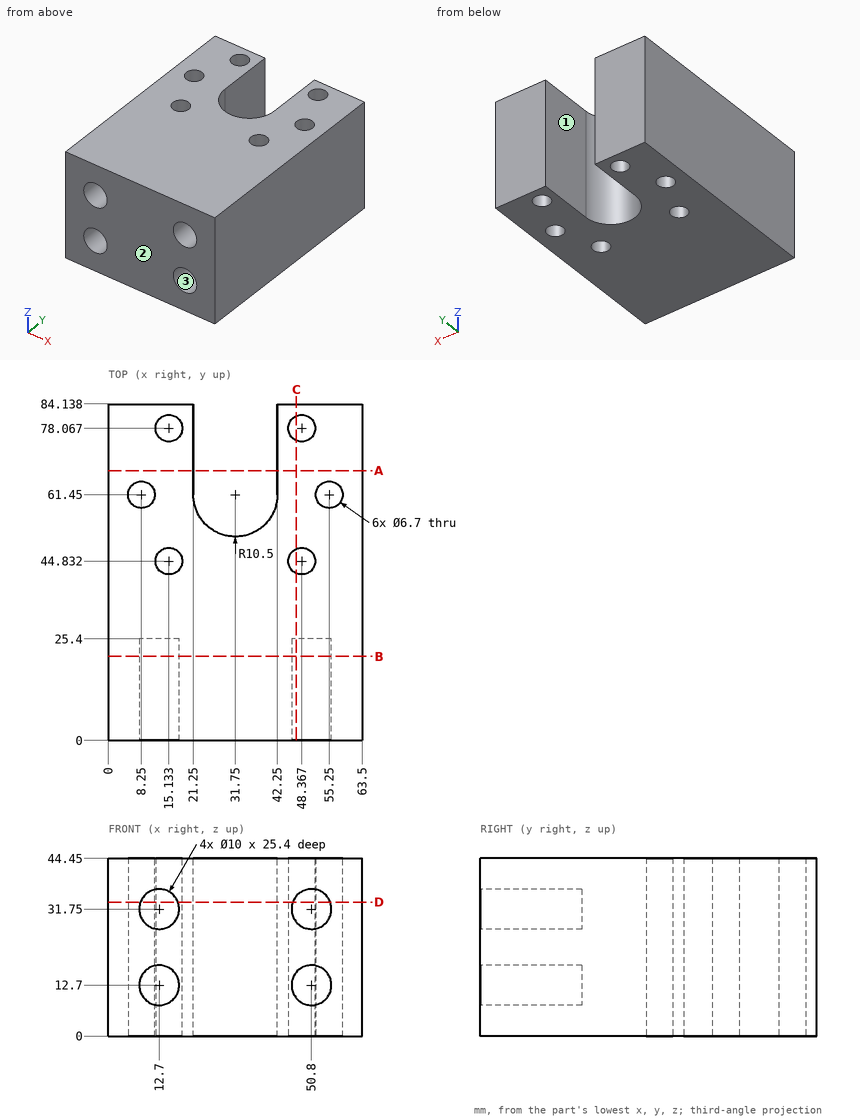
For this review, use the dimensioned drawing (mm, ordinates from the lowest corner) and the shaded views. A direction names the side the tool comes from. Coordinates: 2 decimals unless noted, no trailing zeros. Order: outer loops, then holes, each group sorted by start corner. A loop starts at its lowest first (then second) coordinate and runs counter-clockwise, first axis right, second up. Notation, with made-up numbers: (23, 46.25) - (28, 46.25) arc R14 cw to (28, 52.25) - close; hole circle Ø1 at (44, 7.5). An arc over 180 degrees is marked (long way). Answer as a JSON object with one key per item and string values. Group by question number.
1. Clearance check with flat-ended pins moving along their axes: P1, Ø10.5, axis at x = 48.37, y = 44.83, coming from the -Z side; P2, Ø5, axis at x = 51, z = 30, coming from the -Y side. State where each tip first meets the part, or that it passes through.
2. For probe 1 along Z at (x, y) = (12.7, 8.25); probe 2 along X at (y, z) = (63, 40); probe 3 along Y at (x, z) = (55.5, 3), list the stretches that pass through material, from the lowest coordinate up.
3. We need section B-B on y = 21. State the section outline as (x, z) points, then the cut area to 3 significant figures.
4. We need section C-C on x = 47. Give the number of separate pieces and of enclosed holes in the cut face, then the cut area to 3 significant figures.
5. We need section D-D on z = 33.5. State the section outline as (x, y) points.
6. We need section A-A on y = 67.5. State the section outline as (x, z) points.
7. For the marked faces 1, 2 and 3, list the 3-axis set-ups (+Z, -Z, +X, -X, +Y, -Y) from which the entire face can be reached by the end or side of a thin tool; tool diameter is ignored.
Final values:
{
 "1": {"P1": "z = 0", "P2": "y = 25.4"},
 "2": {"probe 1": "0 to 7.7, 17.7 to 26.75, 36.75 to 44.45", "probe 2": "0 to 5.28, 11.22 to 21.25, 42.25 to 52.28, 58.22 to 63.5", "probe 3": "0 to 58.11, 64.79 to 84.14"},
 "3": {"outline": "(0, 0) - (63.5, 0) - (63.5, 44.45) - (0, 44.45) - close; hole circle Ø10 at (12.7, 12.7); hole circle Ø10 at (12.7, 31.75); hole circle Ø10 at (50.8, 12.7); hole circle Ø10 at (50.8, 31.75)", "area": "2,510 mm²"},
 "4": {"separate pieces": "3", "enclosed holes": "0", "area": "2,870 mm²"},
 "5": {"outline": "(0, 0) - (8.02, 0) - (8.02, 25.4) - (17.38, 25.4) - (17.38, 0) - (46.12, 0) - (46.12, 25.4) - (55.48, 25.4) - (55.48, 0) - (63.5, 0) - (63.5, 84.14) - (42.25, 84.14) - (42.25, 61.45) arc R10.5 cw to (21.25, 61.45) - (21.25, 84.14) - (0, 84.14) - close; hole circle Ø6.7 at (8.25, 61.45); hole circle Ø6.7 at (15.13, 44.83); hole circle Ø6.7 at (15.13, 78.07); hole circle Ø6.7 at (48.37, 44.83); hole circle Ø6.7 at (48.37, 78.07); hole circle Ø6.7 at (55.25, 61.45)"},
 "6": {"outline": "(0, 0) - (21.25, 0) - (21.25, 44.45) - (0, 44.45) - close; (42.25, 0) - (63.5, 0) - (63.5, 44.45) - (42.25, 44.45) - close"},
 "7": {"face 1": "+Z, -Z, +Y", "face 2": "+Z, -Z, +X, -X, -Y", "face 3": "-Y"}
}
